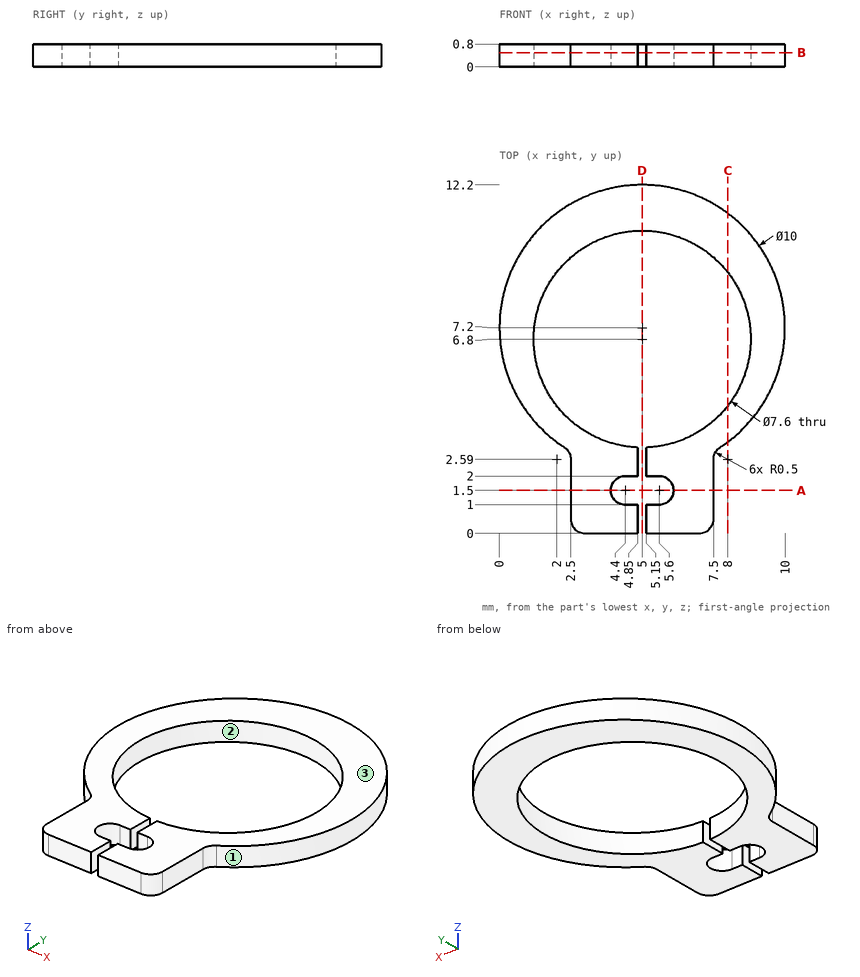
Job drawing, mm, ordinate dimensions from the low corner. One solid piece. Round coordinates to 2 decimals unless told otherwise and drop trailing zeros. Order: outer loops, then holes, each group sorted by start corner. A loop starts at its lowest first (then second) coordinate and runs counter-clockwise, first axis right, second up. Notation, with made-up numbers: (33, 4.25) - (39, 4.25) arc R13 cw to (39, 15.25) - close; hole circle Ø7 at (0.5, 28). An arc over 180 degrees is marked (long way). Use CSV: the item, a comma, the result in double quotes. Start each with the question number.
1) Saw through at D-D (x = 5). List the corners of the cut face in (y, z), and give its area (3 significant figures).
2) Saw through at C-C (x = 8). List the corners of the cut face in (y, z).
3) Two-plate mould, pull along Y, no slides. Class the marked faces 1, 2 and 3: pulls with the +Y half, pulls with the -Y half, needs draft (parallel to the pull), parting line crosses it, or undercut.
4) Wall check: L1, parallel to Y at x = 5.75, z = 0.6 (1 decimal); L2, parallel to Y at x = 3.5, z = 0.55; L3, parallel to X at y = 6.8, z = 0.2. Give the ranges that are in metal, low to high. Write a range as [from, to].
5) Saw through at B-B (z = 0.5). List the corners of the cut face in (x, y).
6) Saw through at A-A (y = 1.5). List the corners of the cut face in (x, z).
Values follow:
1,outline,"(10.6, 0) - (12.2, 0) - (12.2, 0.8) - (10.6, 0.8) - close"
1,area,"1.28 mm2"
2,outline,"(3.2, 0) - (4.47, 0) - (4.47, 0.8) - (3.2, 0.8) - close; (9.13, 0) - (11.2, 0) - (11.2, 0.8) - (9.13, 0.8) - close"
3,face 1,"parting line crosses it"
3,face 2,"undercut"
3,face 3,"needs draft"
4,L1,"y = [0, 1], [2, 3.1], [10.5, 12.1]"
4,L2,"y = [0, 3.31], [10.29, 11.97]"
4,L3,"x = [0.02, 1.2], [8.8, 9.98]"
5,outline,"(2.27, 3.01) arc R0.5 cw to (2.5, 2.59) - (2.5, 0.5) arc R0.5 ccw to (3, 0) - (4.85, 0) - (4.85, 1) - (4.4, 1) arc R0.5 cw to (4.4, 2) - (4.85, 2) - (4.85, 3) arc R3.8 cw (long way) to (5.15, 3) - (5.15, 2) - (5.6, 2) arc R0.5 cw to (5.6, 1) - (5.15, 1) - (5.15, 0) - (7, 0) arc R0.5 ccw to (7.5, 0.5) - (7.5, 2.59) arc R0.5 cw to (7.73, 3.01) arc R5 ccw (long way) to start"
6,outline,"(2.5, 0) - (3.9, 0) - (3.9, 0.8) - (2.5, 0.8) - close; (6.1, 0) - (7.5, 0) - (7.5, 0.8) - (6.1, 0.8) - close"
